Source: CAD feature listing. Evaluate the final solid. Frame: model axes, mm. A direction names the side the tool comes from. Coordinates: 2 decimals unless noted, no trailing zeros. Loops run counter-clockwise (first coordinate to the right, second up) from the corner with the lowest first, then second, coordinate; pieces in that order, holes last.
Item 1: Pull-direction query (Y, two-part tool) for faces 4 (the cylindrical face through (-7.441, 15.815, -11.218)), 5 (the flat face through (0, 77, 3.175)), 6 (the flat face through (5, 56, 132.397)); classes: +Y half, -Y half, draft (parallel to the pull), parting line (faces both ways), or undercut.
Item 2: Pin query (flat end, axial travel): pin 1 Ø0.9 at (y, z) = (79, 2.5) entering from -X; pin 2 Ø4.5 at (x, y) = (-1, 78) entering from -Z (3 decimals); pin 3 Ø3 at (y, z) = (78, 1.5) entering from +X. Return the tip coordinate at first contact, or that it passes through.
Item 3: Reachability of faces 1 (the flat face through (-8.89, 26, -9)), 2 (the cylindrical face through (2.612, 40.938, 95.052)), 3 (the flat face through (-15, 8, 3.175)) from +Z, -Z, +X, -X, +Y, -Y: full face, straight path, thin tool, end or side. Return the list, or none.
Item 4: Section query C-C, the plane x = 0. State how many separate pieces and enclosed holes the cut face has, then the cut area to 3 significant figures.
Item 5: Section query A-A, the plane z = 114. Return the cut outline in (x, y).
Item 6: Section query D-D, the plane z = 150.5. Return the cut outline in (x, y), then the cut area to 3 significant figures.
Item 7: Section query B-B, the plane y = 70. Return the cut outline in (x, z), then the cut area to 3 significant figures.
Item 8: Line query: probe 1 along Z at (x, y) = (-1, 58.5); probe 2 along Z at (x, y) = (-5.5, 65); probe 3 along Y at (x, z) = (5, 54). Output: solid intervals per line, ascending.
```python
from build123d import *

# Parameters (mm, degrees)
BOSS_EXTRUDE1_DEPTH                      = 58.7375
SKETCH2_R                                = 20.066
BOSS_EXTRUDE2_DEPTH                      = 73.66
EDIT_LENGTH_HERE_HOVER_FOR_COMMENT_DEPTH = 113.792
SKETCH4_R                                = 9.9822
BOSS_EXTRUDE4_DEPTH                      = 25.4
BOSS_EXTRUDE5_DEPTH                      = 20.6502
CUT_EXTRUDE3_DEPTH                       = 217.231560923
CUT_EXTRUDE3_DEPTH_BACK                  = 217.231560923
SKETCH6_R                                = 3.3782
FILLET1_R                                = 2.54
FILLET2_R                                = 0.508
CUT_EXTRUDE5_DEPTH                       = 3.81
SKETCH8_R                                = 6.5405
BOSS_EXTRUDE6_DEPTH                      = 4.445
FILLET3_R                                = 0.0254
BOSS_EXTRUDE7_START                      = -12.7
BOSS_EXTRUDE7_DEPTH                      = 12.7
SKETCH10_R                               = 2.54
BOSS_EXTRUDE8_DEPTH                      = 0.635


with BuildPart() as part:
    # Sketch1 → Boss-Extrude1 (new body)
    with BuildSketch(Plane.XY):
        with BuildLine():
            Line((-12.7, 0), (12.7, 0))
            Line((12.7, 0), (20.955, 6.35))
            Line((20.955, 6.35), (20.955, 60.833))
            ThreePointArc((20.955, 60.833), (0, 81.788), (-20.955, 60.833))
            Line((-20.955, 60.833), (-20.955, 6.35))
            Line((-20.955, 6.35), (-12.7, 0))
        make_face()
    extrude(amount=BOSS_EXTRUDE1_DEPTH)

    # Sketch2 → Boss-Extrude2 (add)
    with BuildSketch(Plane.XY.offset(58.7375)):
        with Locations(Location((0, 60.833, 0), (0, 0, 180))):
            Circle(SKETCH2_R)
    extrude(amount=BOSS_EXTRUDE2_DEPTH)

    # Sketch3 → EDIT_LENGTH_HERE (hover for comment) (add)
    with BuildSketch(Plane.XY.offset(58.7375)):
        with BuildLine():
            Line((-14.88814822, 20.042680112), (-10.996912775, 1.5621))
            Line((-10.996912775, 1.5621), (10.996912775, 1.5621))
            Line((10.996912775, 1.5621), (14.88814822, 20.042680112))
            ThreePointArc((14.88814822, 20.042680112), (0, 38.3921), (-14.88814822, 20.042680112))
        make_face()
    extrude(amount=EDIT_LENGTH_HERE_HOVER_FOR_COMMENT_DEPTH)

    # Sketch4 → Boss-Extrude4 (add)
    with BuildSketch(Plane.XY.offset(172.5295)):
        with Locations((0, 23.1775)):
            Circle(SKETCH4_R)
    extrude(amount=BOSS_EXTRUDE4_DEPTH)

    # Sketch5 → Boss-Extrude5 (add)
    with BuildSketch(Plane(origin=(0, 0, 0), x_dir=(-1, 0, 0), z_dir=(0, 0, -1))):
        with BuildLine():
            Line((-3.81, 32.0675), (3.81, 32.0675))
            ThreePointArc((3.81, 32.0675), (7.402102448, 30.579602448), (8.89, 26.9875))
            Line((8.89, 26.9875), (8.89, 19.3675))
            ThreePointArc((8.89, 19.3675), (7.402102448, 15.775397552), (3.81, 14.2875))
            Line((3.81, 14.2875), (-3.81, 14.2875))
            ThreePointArc((-3.81, 14.2875), (-7.402102448, 15.775397552), (-8.89, 19.3675))
            Line((-8.89, 19.3675), (-8.89, 26.9875))
            ThreePointArc((-8.89, 26.9875), (-7.402102448, 30.579602448), (-3.81, 32.0675))
        make_face()
    extrude(amount=BOSS_EXTRUDE5_DEPTH)

    # Sketch6 → Cut-Extrude3 (cut, two sides: drawn at the far end of the back side and taken through both)
    with BuildSketch(Plane(origin=(8.89, 0, 0), x_dir=(0, 0, -1), z_dir=(1, 0, 0)).offset(-CUT_EXTRUDE3_DEPTH_BACK)):
        with Locations((11.90625, 23.1775)):
            Circle(SKETCH6_R)
        with Locations(Location((-188.4045, 23.1775, 0), (0, 0, 179.999999986))):
            Circle(SKETCH6_R)
    extrude(amount=CUT_EXTRUDE3_DEPTH + CUT_EXTRUDE3_DEPTH_BACK, mode=Mode.SUBTRACT)

    # Fillet1
    fillet1_edges = [part.edges().sort_by_distance(p)[0] for p in [
        (7.402102448, 15.775397552, 0),
        (0, 14.2875, 0),
        (-7.402102448, 15.775397552, 0),
        (-8.89, 23.1775, 0),
        (-7.402102448, 30.579602448, 0),
        (0, 32.0675, 0),
        (7.402102448, 30.579602448, 0),
        (8.89, 23.1775, 0),
    ]]
    fillet(fillet1_edges, radius=FILLET1_R)

    # Fillet2
    fillet2_edges = [part.edges().sort_by_distance(p)[0] for p in [
        (7.402102448, 15.775397552, -20.6502),
        (0, 14.2875, -20.6502),
        (-7.402102448, 15.775397552, -20.6502),
        (-8.89, 23.1775, -20.6502),
        (-7.402102448, 30.579602448, -20.6502),
        (0, 32.0675, -20.6502),
        (7.402102448, 30.579602448, -20.6502),
        (8.89, 23.1775, -20.6502),
    ]]
    fillet(fillet2_edges, radius=FILLET2_R)

    # Sketch7 → Cut-Extrude5 (cut)
    with BuildSketch(Plane(origin=(0, 0, 0), x_dir=(-1, 0, 0), z_dir=(0, 0, -1))):
        with BuildLine():
            Line((-4.1275, 80.068311519), (-4.1275, 77.089))
            ThreePointArc((-4.1275, 77.089), (0, 72.9615), (4.1275, 77.089))
            Line((4.1275, 77.089), (4.1275, 79.978628931))
            ThreePointArc((4.1275, 79.978628931), (4.367379625, 80.721429048), (4.996400809, 81.183626623))
            ThreePointArc((4.996400809, 81.183626623), (0.071861599, 81.787876781), (-4.856706104, 81.217416372))
            ThreePointArc((-4.856706104, 81.217416372), (-4.325187488, 80.748786262), (-4.1275, 80.068311519))
        make_face()
        with BuildLine():
            ThreePointArc((-19.685, 11.610879552), (-20.583025612, 11.98285394), (-20.955, 12.880879552))
            Line((-20.955, 12.880879552), (-20.955, 6.35))
            Line((-20.955, 6.35), (-13.042377801, 0.26336754))
            ThreePointArc((-13.042377801, 0.26336754), (-13.507857108, 0.994743297), (-13.395607029, 1.854383572))
            Line((-13.395607029, 1.854383572), (-11.222314297, 6.047728836))
            ThreePointArc((-11.222314297, 6.047728836), (-11.349573436, 9.780348644), (-14.605, 11.610879552))
            Line((-14.605, 11.610879552), (-19.685, 11.610879552))
        make_face()
        with BuildLine():
            Line((20.955, 6.35), (20.955, 12.880879552))
            ThreePointArc((20.955, 12.880879552), (20.583025612, 11.98285394), (19.685, 11.610879552))
            Line((19.685, 11.610879552), (14.605, 11.610879552))
            ThreePointArc((14.605, 11.610879552), (11.203032914, 9.51631534), (11.541558483, 5.535614431))
            Line((11.541558483, 5.535614431), (13.402295436, 1.841293477))
            ThreePointArc((13.402295436, 1.841293477), (13.506243345, 0.987572709), (13.042377827, 0.263367559))
            Line((13.042377827, 0.263367559), (20.955, 6.35))
        make_face()
    extrude(amount=-CUT_EXTRUDE5_DEPTH, mode=Mode.SUBTRACT)

    # Sketch8 → Boss-Extrude6 (add)
    with BuildSketch(Plane.XY.offset(132.3975)):
        with Locations((0, 60.833)):
            Circle(SKETCH8_R)
    extrude(amount=BOSS_EXTRUDE6_DEPTH)

    # Fillet3
    fillet3_edges = [part.edges().sort_by_distance(p)[0] for p in [
        (-6.5405, 60.833, 132.3975),
        (-6.5405, 60.833, 136.8425),
    ]]
    fillet(fillet3_edges, radius=FILLET3_R)

    # Sketch9 → Boss-Extrude7 (add)
    with BuildSketch(Plane.XY.offset(172.5295).offset(BOSS_EXTRUDE7_START)):
        with BuildLine():
            Line((-11.017521545, 1.5367), (11.017521545, 1.5367))
            Line((11.017521545, 1.5367), (14.913003226, 20.03744669))
            ThreePointArc((14.913003226, 20.03744669), (0, 38.4175), (-14.913003226, 20.03744669))
            Line((-14.913003226, 20.03744669), (-11.017521545, 1.5367))
        make_face()
        with BuildLine():
            Line((10.996912775, 1.5621), (14.88814822, 20.042680112))
            ThreePointArc((14.88814822, 20.042680112), (0, 38.3921), (-14.88814822, 20.042680112))
            Line((-14.88814822, 20.042680112), (-10.996912775, 1.5621))
            Line((-10.996912775, 1.5621), (10.996912775, 1.5621))
        make_face(mode=Mode.SUBTRACT)
    extrude(amount=BOSS_EXTRUDE7_DEPTH)

    # Sketch10 → Boss-Extrude8 (add)
    with BuildSketch(Plane(origin=(0, 0, 3.81), x_dir=(-1, 0, 0), z_dir=(0, 0, -1))):
        with Locations((0, 77.089)):
            Circle(SKETCH10_R)
        with Locations((-14.605, 7.800879552)):
            Circle(SKETCH10_R)
        with Locations((14.605, 7.800879552)):
            Circle(SKETCH10_R)
    extrude(amount=BOSS_EXTRUDE8_DEPTH)


solid = part.part
```
Verdict:
1. face 4: -Y half
1. face 5: draft
1. face 6: undercut
2. pin 1: stops at x = -11.19
2. pin 2: stops at z = 3.175
2. pin 3: stops at x = 13.92
3. face 1: -Z, -X, +Y, -Y
3. face 2: +Z
3. face 3: -Z, -X
4. separate pieces: 1
4. enclosed holes: 2
4. area: 12,800 mm2
5. outline: circle Ø40.13 at (0, 60.83); (-14.89, 20.04) - (-11, 1.56) - (11, 1.56) - (14.89, 20.04) arc R15.21 ccw (long way) to start
6. outline: (-14.89, 20.04) - (-11, 1.56) - (11, 1.56) - (14.89, 20.04) arc R15.21 ccw (long way) to start
6. area: 937 mm2
7. outline: (-18.84, 0) - (18.84, 0) - (18.84, 58.74) - (17.85, 58.74) - (17.85, 132.4) - (-17.85, 132.4) - (-17.85, 58.74) - (-18.84, 58.74) - close
7. area: 4,840 mm2
8. probe 1: z = 0 to 136.84
8. probe 2: z = 0 to 132.4
8. probe 3: y = 0 to 81.18
